```python
from build123d import *

# Parameters (mm, degrees)
SKETCH1_W               = 13
SKETCH1_H               = 8
BOSS_EXTRUDE1_DEPTH     = 3
CUT_EXTRUDE1_DEPTH      = 16.556349186
CUT_EXTRUDE1_DEPTH_BACK = 16.556349186
CUT_EXTRUDE2_DEPTH      = 16.556349186
CUT_EXTRUDE2_DEPTH_BACK = 16.556349186
SKETCH4_R               = 1.75
CUT_EXTRUDE3_DEPTH      = 0.4
SKETCH5_W               = 8
SKETCH5_H               = 1.1
BOSS_EXTRUDE2_DEPTH     = 2
FILLET1_R               = 4
CUT_EXTRUDE4_DEPTH      = 0.4


with BuildPart() as part:
    # Sketch1 → Boss-Extrude1 (new body)
    with BuildSketch(Plane(origin=(0, 0, 0), x_dir=(1, 0, 0), z_dir=(0, 1, 0))):
        with Locations((6.5, 4)):
            Rectangle(SKETCH1_W, SKETCH1_H)
    extrude(amount=BOSS_EXTRUDE1_DEPTH)

    # Sketch2 → Cut-Extrude1 (cut, two sides: drawn at the far end of the back side and taken through both)
    with BuildSketch(Plane.XY.offset(-CUT_EXTRUDE1_DEPTH_BACK)):
        Polygon((0, 0), (0.6, 3), (0, 3), align=None)
        Polygon((13, 0), (12.4, 3), (13, 3), align=None)
    extrude(amount=CUT_EXTRUDE1_DEPTH + CUT_EXTRUDE1_DEPTH_BACK, mode=Mode.SUBTRACT)

    # Sketch3 → Cut-Extrude2 (cut, two sides: drawn at the far end of the back side and taken through both)
    with BuildSketch(Plane(origin=(0, 0, 0), x_dir=(0, 0, -1), z_dir=(1, 0, 0)).offset(-CUT_EXTRUDE2_DEPTH_BACK)):
        Polygon((0, 0), (0.6, 3), (0, 3), align=None)
        Polygon((8, 3), (7.4, 3), (8, 0), align=None)
    extrude(amount=CUT_EXTRUDE2_DEPTH + CUT_EXTRUDE2_DEPTH_BACK, mode=Mode.SUBTRACT)

    # Sketch4 → Cut-Extrude3 (cut)
    with BuildSketch(Plane.XZ):
        with Locations(Location((6.50000125, -3.75, 0), (0, 0, 270))):
            Circle(SKETCH4_R)
    extrude(amount=-CUT_EXTRUDE3_DEPTH, mode=Mode.SUBTRACT)

    # Sketch5 → Boss-Extrude2 (add)
    with BuildSketch(Plane.XZ):
        with Locations((6.500011, -7.45)):
            Rectangle(SKETCH5_W, SKETCH5_H)
    extrude(amount=BOSS_EXTRUDE2_DEPTH)

    # Fillet1
    # the kernel refuses this fillet: 4 mm, written as the material it takes off along each edge
    with BuildSketch(Plane(origin=(10.500011, -2, -16.660254038), x_dir=(0, 1, 0), z_dir=(0, 0, 1)), Plane(origin=(2.500011, -2, 1.760254038), x_dir=(0, 1, 0), z_dir=(0, 0, -1))) as fillet1_piece_1:
        with BuildLine():
            CenterArc((4, 3.464101615), FILLET1_R, 180, 60)
            Line((0, 3.464101615), (-0.08, 3.464101615))
            Line((-0.08, 3.464101615), (-0.08, 0))
            Line((-0.08, 0), (0, -0.08))
            ThreePointArc((0, -0.08), (1, -0.08), (1.96, -0.069282032))
            Line((1.96, -0.069282032), (2, 0))
        make_face()
    extrude(amount=18.420508076, mode=Mode.SUBTRACT)

    # Sketch6 → Cut-Extrude4 (cut)
    # profile 1 of 3: a face of its own
    with BuildSketch(Plane(origin=(0, 3, 0), x_dir=(1, 0, 0), z_dir=(0, 1, 0))):
        Polygon((5.356583629, 2.605681315), (4.744804782, 2.605681315), (4.491799975, 3.297989008), (3.340357667, 3.297989008), (3.087352859, 2.605681315), (2.471968244, 2.605681315), (3.605982667, 5.605681315), (4.217160552, 5.605681315), align=None)
        Polygon((4.308506705, 3.797989008), (3.914275936, 4.874912084), (3.52124709, 3.797989008), align=None, mode=Mode.SUBTRACT)
    # profile 2 of 3: a face of its own
    with BuildSketch(Plane(origin=(0, 3, 0), x_dir=(1, 0, 0), z_dir=(0, 1, 0))):
        Polygon((5.664275936, 2.605681315), (5.664275936, 5.605681315), (6.241199013, 5.605681315), (6.241199013, 3.105681315), (7.779660552, 3.105681315), (7.779660552, 2.605681315), align=None)
    # profile 3 of 3: a face of its own
    with BuildSketch(Plane(origin=(0, 3, 0), x_dir=(1, 0, 0), z_dir=(0, 1, 0))):
        Polygon((8.895045167, 2.605681315), (8.895045167, 5.105681315), (8.010429782, 5.105681315), (8.010429782, 5.605681315), (10.356583629, 5.605681315), (10.356583629, 5.105681315), (9.471968244, 5.105681315), (9.471968244, 2.605681315), align=None)
    extrude(amount=-CUT_EXTRUDE4_DEPTH, mode=Mode.SUBTRACT)


solid = part.part
```
Input: part model. Units: mm. Frame: model coordinates. A direction names the side the tool comes from. Give positions to 0.01 mm unless a question says otherwise; leave off trailing zeros. Order: outer loops, then holes, each group sorted by start corner. A loop starts at its lowest first (then second) coordinate and runs counter-clockwise, first axis right, second up. Notation, with made-up numbers: (58, 58) - (104, 58) arc R15 cw to (104, 77) - close; hole circle Ø5 at (-16, 12.5). An arc over 180 degrees is marked (long way). Put each result on its own line as item: value.
Item 1: Section query D-D, the plane z = -2.25. Return loops of the section in (x, y).
Found:
outline: (0, 0) - (5.6, 0) - (5.6, 0.4) - (7.4, 0.4) - (7.4, 0) - (13, 0) - (12.4, 3) - (0.6, 3) - close
Item 2: Section query B-B, the plane x = 6.75. Return loops of the section in (y, z).
Found:
outline: (-2, -8) - (0, -8) - (3, -7.4) - (3, -3.11) - (2.6, -3.11) - (2.6, -2.61) - (3, -2.61) - (3, -0.6) - (0, 0) - (0, -2.02) - (0.4, -2.02) - (0.4, -5.48) - (0, -5.48) - (0, -6.9) - (-2, -6.9) - close
Item 3: Ray query, L1, parallel to Z at x = 8, y = -0.75; L2, parallel to Y at x = 4, z = -1.5; L3, parallel to X at y = 0.1, z = -3.75. Return the intervals inside material, ascending. Write a range as from..to.
Found:
L1: z = -8..-6.9
L2: y = 0..3
L3: x = 0.02..4.75, 8.25..12.98
Item 4: Contact query for a flat-ended pin moving along its axis: pin 1 (1.6 mm diameter, centred on x = 5.5, y = -1, fed in from +Z). Output: stop coordinate, or through.
Found:
pin 1: stops at z = -6.9
Item 5: Section query A-A, the plane z = -7.25. Return loops of the section in (x, y), then the cut area to 3 significant figures.
Found:
outline: (0, 0) - (2.5, 0) arc R4 ccw to (5.96, -2) - (7.04, -2) arc R4 ccw to (10.5, 0) - (13, 0) - (12.4, 3) - (0.6, 3) - close
area: 49.2 mm^2
Item 6: Section query C-C, the plane y = 2.45. Return loops of the section in (x, z).
Found:
outline: (0.49, -7.51) - (12.51, -7.51) - (12.51, -0.49) - (0.49, -0.49) - close
Item 7: Access query for faces 5 (the flat face through (3.03, 2.8, -4.08)), 6 (the flat face through (7, 0.4, -4)), 7 (the cylindrical face through (3.99, -1.48, -7.44)). Directions: +Z, -Z, +X, -X, +Y, -Y. A direction counts if a zero-diameter tool reaches every point of the face in a straight line with its end or side. Return the directions, or none.
Found:
face 5: +Y
face 6: -Y
face 7: +Z, -Z, -X, -Y
Item 8: Draft query along X for faces 1 (the flat face through (9.2, 2.6, -4.5)), 2 (the flat face through (6, -1, -6.9)), 3 (the flat face through (6, 2.6, -4)), 4 (the flat face through (12.7, 1.5, -4.1)). Return one class per face: +X half, -X half, draft (parallel to the pull), parting line (faces both ways), or undercut.
Found:
face 1: undercut
face 2: draft
face 3: undercut
face 4: +X half
